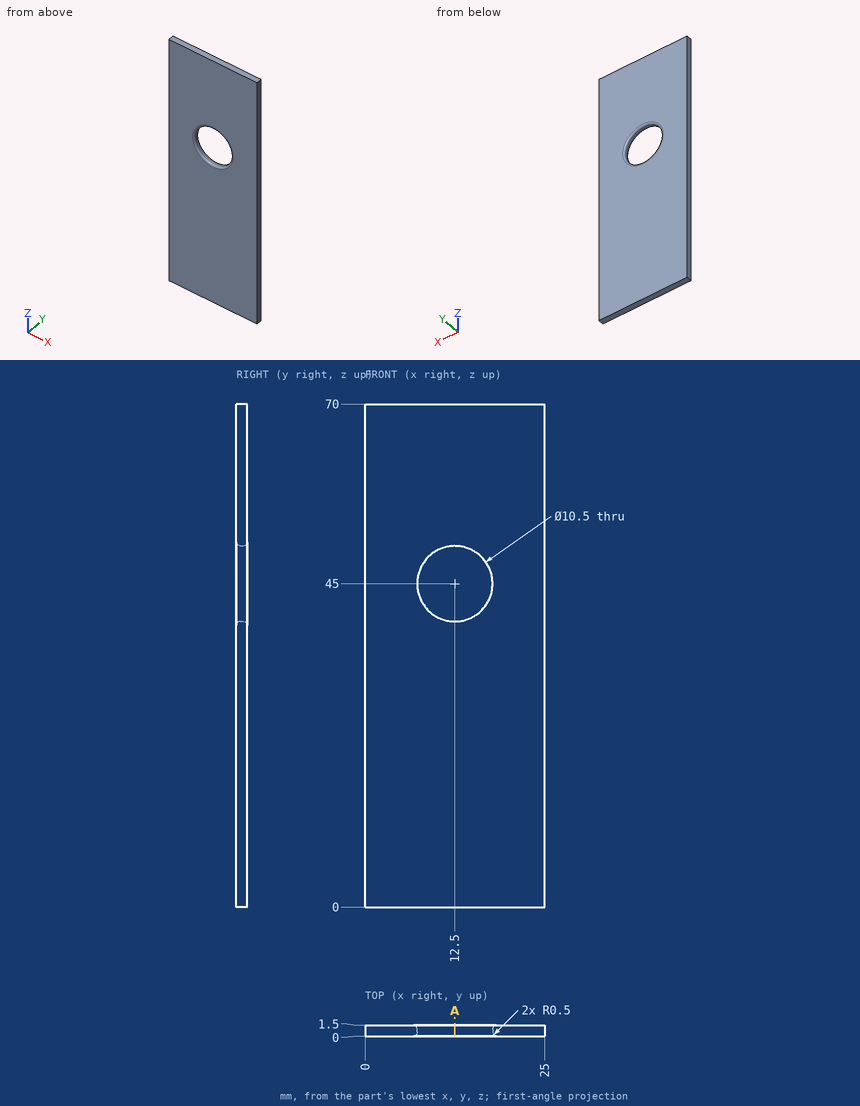
Geometry check sheet. Reference: drawing and pictorial views, mm from the part's lowest x, y, z. Give positions to 0.01 mm unless a question says otherwise; leave off trailing zeros. Order: outer loops, then holes, each group sorted by start corner. A loop starts at its lowest first (then second) coordinate and runs counter-clockwise, first axis right, second up. Notation, with made-up numbers: M 88,31 L 118,31 A14 cw 118,39 Z; hole C 56,60.5 d7. An arc over 180 degrees is marked long. Answer as CSV lines item,"result". Start each with the question number.
Item 1: Gauge pin test, flat end, axial feed: P1, Ø8.5, axis at x = 12.5, z = 45, coming from the -Y side. Record the tip position at first contact, or that the pin passes through.
Item 2: Thickness scan on line 1 (Z direction, x = 12.5, y = 0.65); line 2 (Z direction, x = 16, y = 0.15); line 3 (Y direction, x = 7.5, z = 47.5). Record the ranges inside material, lowest first. Write a range as [from, to].
Item 3: Cross-section at A-A on x = 12.5. Enter the section's corners in (y, z).
Established:
1,P1,"passes through"
2,line 1,"z = [0, 39.75], [50.25, 70]"
2,line 2,"z = [0, 40.9], [49.1, 70]"
2,line 3,"y = [0.03, 1.47]"
3,outline,"M 0,0 L 1.5,0 L 1.5,39.25 A0.5 ccw 1,39.75 L 0.5,39.75 A0.5 ccw 0,39.25 Z; M 0,50.75 A0.5 ccw 0.5,50.25 L 1,50.25 A0.5 ccw 1.5,50.75 L 1.5,70 L 0,70 Z"
